Could you check a few things on this drawing? It's one solid part, dimensions in mm from its lowest x, y, z. A direction names the side the tool comes from. Coordinates: 2 decimals unless noted, no trailing zeros. Order: outer loops, then holes, each group sorted by start corner. A loop starts at its lowest first (then second) coordinate and runs counter-clockwise, first axis right, second up. Notation, with made-up numbers: (75, -14.75) -> (107, -14.75) arc R22 cw to (107, 17.25) -> close; hole circle Ø9 at (-39, 3). An arc over 180 degrees is marked (long way). Answer as CSV lines item,"result".
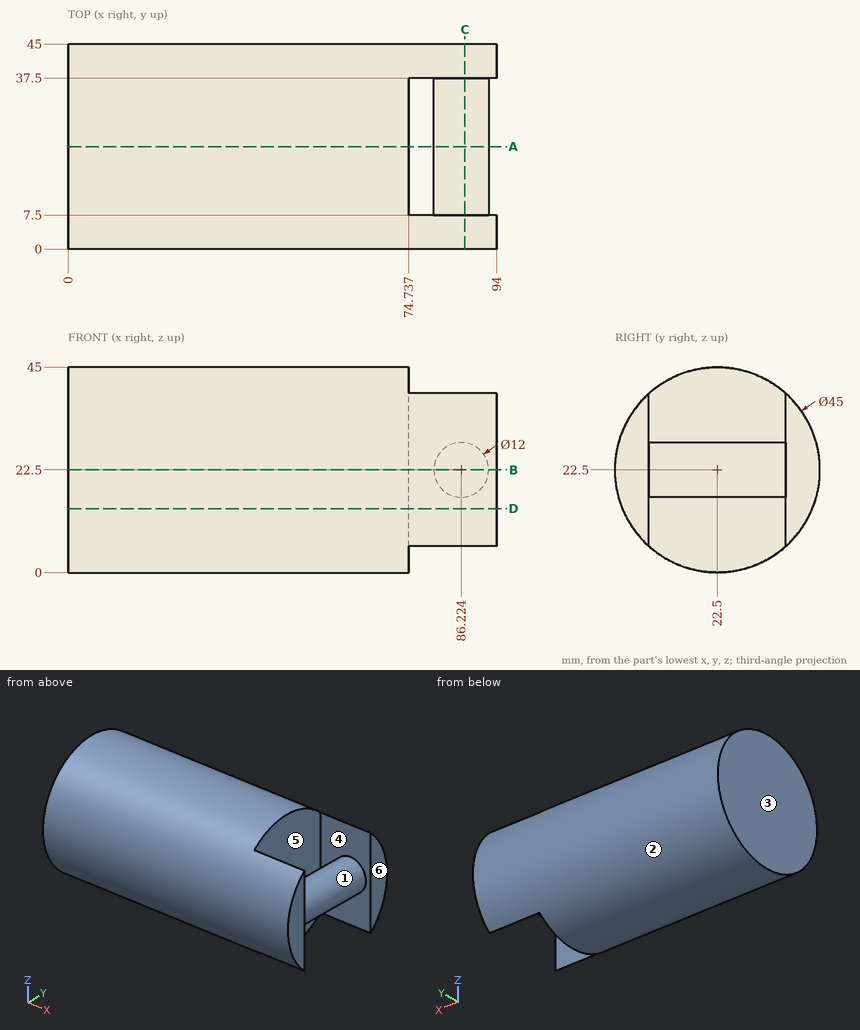
Q1. Imagine slicing it at B-B (z = 22.5). List the corners of the cut face in (x, y) for me (1 decimal).
Solution:
outline,"(0, 0) -> (94, 0) -> (94, 7.5) -> (92.2, 7.5) -> (92.2, 37.5) -> (94, 37.5) -> (94, 45) -> (0, 45) -> close; hole (74.7, 7.5) -> (80.2, 7.5) -> (80.2, 37.5) -> (74.7, 37.5) -> close"
Q2. Which directions (+Z, -Z, +X, -X, +Y, -Y) give clear straight access to the entire face, cutting with the end or side of a thin tool? Please do the marked faces 4, 5 and 6.
Solution:
face 4,"none"
face 5,"+Z, -Z"
face 6,"+Z, -Z, +X, +Y, -Y"
Q3. We'd pull the mould along X, two halves only. Please class the marked faces 1, 2 and 3: pulls with the +X half, pulls with the -X half, needs draft (parallel to the pull), parting line crosses it, or undercut.
Solution:
face 1,"undercut"
face 2,"needs draft"
face 3,"pulls with the -X half"
Q4. Imagine slicing it at A-A (y = 22.5). List the corners of the cut face in (x, z) for me (1 decimal), and give its area (3 significant figures).
Solution:
outline,"(0, 0) -> (74.7, 0) -> (74.7, 45) -> (0, 45) -> close; circle Ø12 at (86.2, 22.5)"
area,"3,480 mm2"
Q5. For P1, Ø6, axis at x = 52, z = 14, coming from the -Y side; P2, Ø9.5, axis at x = 88, z = 15, coming from the +Y side; P3, Ø8, axis at x = 49, z = 30.5, coming from the -Y side, each with a flat end and sliding along its axis, tell me the tip position at first contact or that it passes through.
Solution:
P1,"y = 0.68"
P2,"y = 44.83"
P3,"y = 0.36"
Q6. Imagine slicing it at D-D (z = 14). List the corners of the cut face in (x, y) for me, and give its area (3 significant figures).
Solution:
outline,"(0, 1.67) -> (94, 1.67) -> (94, 7.5) -> (74.74, 7.5) -> (74.74, 37.5) -> (94, 37.5) -> (94, 43.33) -> (0, 43.33) -> close"
area,"3,340 mm2"
Q7. Imagine slicing it at C-C (x = 87). List the corners of the cut face in (y, z) for me.
Solution:
outline,"(7.5, 5.73) -> (7.5, 16.55) -> (37.5, 16.55) -> (37.5, 5.73) arc R22.5 ccw to (37.5, 39.27) -> (37.5, 28.45) -> (7.5, 28.45) -> (7.5, 39.27) arc R22.5 ccw to start"
Q8. If I drill on line 1 (X direction, y = 28.5, z = 23) (1 decimal); line 2 (Z direction, x = 62.5, y = 22.5); line 3 (X direction, y = 19, z = 39), over which ranges is the centre line in solid material (lowest first)?
Solution:
line 1,"0 to 74.7, 80.2 to 92.2"
line 2,"0 to 45"
line 3,"0 to 74.74"
